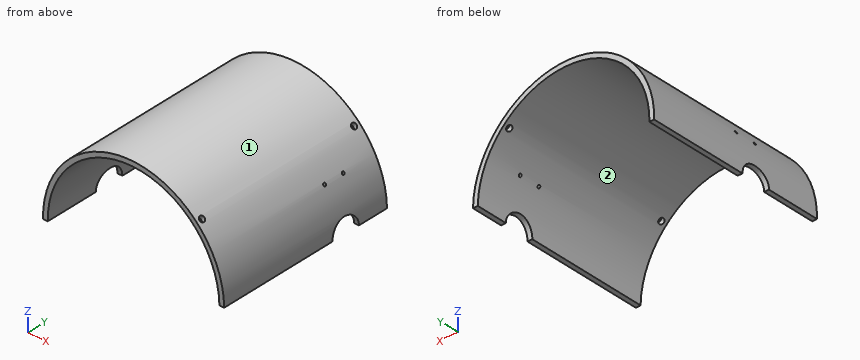
```python
from build123d import *

# Parameters (mm, degrees)
BOSS_EXTRUDE1_DEPTH     = 130.8
SKETCH34_R              = 10.65
CUT_EXTRUDE2_DEPTH      = 157.940740259
SKETCH35_R              = 10.65
CUT_EXTRUDE3_DEPTH      = 157.940740428
CUT_EXTRUDE8_DEPTH      = 132.768470688
CUT_EXTRUDE8_DEPTH_BACK = 132.768470688
SKETCH40_R              = 2
CUT_EXTRUDE9_DEPTH      = 136.886547659
CUT_EXTRUDE9_DEPTH_BACK = 136.886547659
SKETCH41_R              = 2.000000001
SKETCH42_R              = 1
CUT_EXTRUDE10_DEPTH     = 159.175431949
SKETCH43_R              = 1
CUT_EXTRUDE11_DEPTH     = 158.012751408


with BuildPart() as part:
    # Sketch1 → Boss-Extrude1 (new body)
    with BuildSketch(Plane(origin=(0, 0, 0), x_dir=(0.999872775920664, 0, 0.01595092388251422), z_dir=(0, 1, 0))):
        with BuildLine():
            Line((70.372282363, 4.818066557), (66.856282363, 4.818066557))
            ThreePointArc((66.856282363, 4.818066557), (4.002282363, -58.035933443), (-58.851717637, 4.818066557))
            Line((-58.851717637, 4.818066557), (-62.367717637, 4.818066557))
            ThreePointArc((-62.367717637, 4.818066557), (4.002282363, -61.551933443), (70.372282363, 4.818066557))
        make_face()
    extrude(amount=BOSS_EXTRUDE1_DEPTH)

    # Sketch34 → Cut-Extrude2 (cut, through all)
    with BuildSketch(Plane(origin=(4.409550098, 18.583358198, -25.497377904), x_dir=(0.01595092388251443, 0, -0.9998727759206639), z_dir=(0.9998727759206639, 0, 0.01595092388251443))):
        with Locations((-20.746403865, 79.066641802)):
            Circle(SKETCH34_R)
    extrude(amount=CUT_EXTRUDE2_DEPTH, mode=Mode.SUBTRACT)

    # Sketch35 → Cut-Extrude3 (cut, through all)
    with BuildSketch(Plane(origin=(4.409550098, 18.583358198, -25.497377904), x_dir=(0.01595092388251443, 0, -0.9998727759206639), z_dir=(0.9998727759206639, 0, 0.01595092388251443))):
        with Locations((-20.746403865, 30.666641802)):
            Circle(SKETCH35_R)
    extrude(amount=-CUT_EXTRUDE3_DEPTH, mode=Mode.SUBTRACT)

    # Sketch40 → Cut-Extrude8 (cut, two sides: drawn at the far end of the back side and taken through both)
    with BuildSketch(Plane(origin=(3.677708785, 38.899932993, -5.167441514), x_dir=(-0.6958141043149662, 0, -0.7182219240850014), z_dir=(0.7182219240850014, 0, -0.6958141043149662)).offset(-CUT_EXTRUDE8_DEPTH_BACK)):
        with Locations(Location((-0.576184071, 87.550067007, 0), (0, 0, 180))):
            Circle(SKETCH40_R)
        with Locations(Location((-0.576184071, -34.599932993, 0), (0, 0, 180))):
            Circle(SKETCH40_R)
    extrude(amount=CUT_EXTRUDE8_DEPTH + CUT_EXTRUDE8_DEPTH_BACK, mode=Mode.SUBTRACT)

    # Sketch41 → Cut-Extrude9 (cut, two sides: drawn at the far end of the back side and taken through both)
    with BuildSketch(Plane(origin=(8.558168581, 38.899932993, -9.093398931), x_dir=(-0.7182219240850014, 0, 0.6958141043149662), z_dir=(-0.6958141043149662, 0, -0.7182219240850014)).offset(-CUT_EXTRUDE9_DEPTH_BACK)):
        with Locations((6.236989769, 87.550067007)):
            Circle(SKETCH41_R)
        with Locations((6.236989769, -34.599932997)):
            Circle(SKETCH41_R)
    extrude(amount=CUT_EXTRUDE9_DEPTH + CUT_EXTRUDE9_DEPTH_BACK, mode=Mode.SUBTRACT)

    # Sketch42 → Cut-Extrude10 (cut, through all)
    with BuildSketch(Plane(origin=(57.474877903, 38.899932993, 41.409432257), x_dir=(0.7182958266208218, 0, -0.6957378137338163), z_dir=(0.6957378137338163, 0, 0.7182958266208218))):
        with Locations((12.409477286, 66.250067007)):
            Circle(SKETCH42_R)
        with Locations((12.409477286, 51.250067007)):
            Circle(SKETCH42_R)
    extrude(amount=-CUT_EXTRUDE10_DEPTH, mode=Mode.SUBTRACT)

    # Sketch43 → Cut-Extrude11 (cut, through all)
    with BuildSketch(Plane(origin=(-46.82502092, 38.899932993, 43.748332437), x_dir=(0.6957378137338114, 0, 0.7182958266208266), z_dir=(-0.7182958266208266, 0, 0.6957378137338114))):
        with Locations((-18.211184322, 17.850067007)):
            Circle(SKETCH43_R)
        with Locations((-18.211184322, 2.850067007)):
            Circle(SKETCH43_R)
    extrude(amount=-CUT_EXTRUDE11_DEPTH, mode=Mode.SUBTRACT)


solid = part.part
```
For this review, take the finished solid that the model builds, in its own axes (mm). Face numbers are marked on the shaded views. Round coordinates to 2 decimals unless told otherwise and drop trailing zeros. Write each loop counter-clockwise with the first axis right and the second up, starting at its lowest first coordinate (ties: lowest second). Pieces come first, ordered by that corner, then holes. Notation, with made-up numbers: (-3, 80) -> (53, 80) arc R31 cw to (53, 112) -> close; hole circle Ø4 at (-20, -23.75). An arc over 180 degrees is marked (long way). Use one line per item in the form item = value.
Q1. Consider section D-D (x = -24.5). State the section outline as (y, z) points, then the cut area to 3 significant figures.
Resolved:
outline = (0, 51.23) -> (130.8, 51.23) -> (130.8, 55.15) -> (0, 55.15) -> close
area = 513 mm²
Q2. The part is to be moulded in two halves that separate along X. For the marked faces 1 and 2, say which applies: released by +X, released by -X, zero draft, split by the parting line, or undercut.
Resolved:
face_1 = split by the parting line
face_2 = undercut
Q3. Consider section C-C (z = 33.5). State the section outline as (x, y) points.
Resolved:
outline = (-50.16, 0) -> (-45.79, 0) -> (-45.79, 130.8) -> (-50.16, 130.8) -> close; (53.95, 0) -> (58.32, 0) -> (58.32, 130.8) -> (53.95, 130.8) -> close
Q4. To check wall thickness, follow probe 1 along Z at (x, y) = (3, 58); probe 2 along X at (y, z) = (69.5, 27); probe 3 along X at (y, z) = (105, 45). State the ranges of each line that lie inside material, in increasing order. Write a range as from..to.
Resolved:
probe_1 = 58.09..61.61
probe_2 = -54.2..-50.16, 58.32..62.36
probe_3 = -39.85..-34.33, 42.49..48.01
Q5. Consider section A-A (z = 17). State the section outline as (x, y) points, then the cut area to 3 significant figures.
Resolved:
outline = (-58.63, 0) -> (-54.89, 0) -> (-54.89, 130.8) -> (-58.63, 130.8) -> close; (63.05, 0) -> (66.78, 0) -> (66.78, 130.8) -> (63.05, 130.8) -> close
area = 977 mm²
Q6. Clearance check with flat-ended pins moving along their axes: pin 1 Ø5 at (y, z) = (18.5, 30.5) entering from -X; pin 2 Ø3 at (x, y) = (7.5, 66.5) entering from +Z; pin 3 Ø2 at (x, y) = (40, 29.5) entering from +Z. State where each tip first meets the part, or that it passes through.
Resolved:
pin_1 = -53.65
pin_2 = 61.59
pin_3 = 51.69
